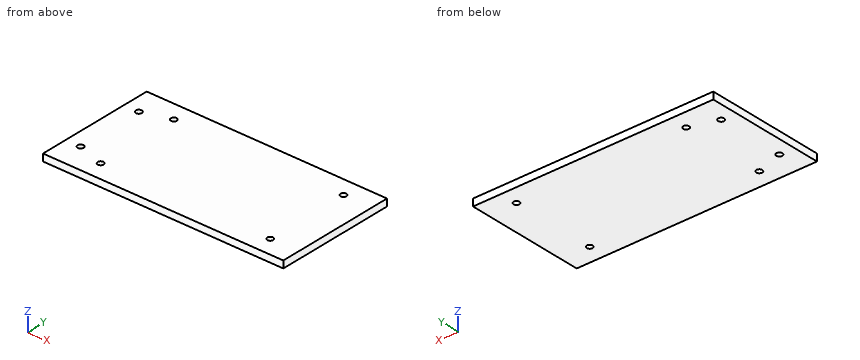
```python
from build123d import *

# Parameters (mm, degrees)
SKETCH1_W           = 85
SKETCH1_H           = 170
SKETCH1_R           = 2.1
BOSS_EXTRUDE1_DEPTH = 5
SKETCH2_R           = 2.15
CUT_EXTRUDE1_DEPTH  = 10
SKETCH3_R           = 2.15
CUT_EXTRUDE2_DEPTH  = 10


with BuildPart() as part:
    # Sketch1 → Boss-Extrude1 (new body)
    with BuildSketch(Plane(origin=(0, 0, 0), x_dir=(0, 1, 0), z_dir=(0, 0, 1))):
        Rectangle(SKETCH1_W, SKETCH1_H)
        with Locations(Location((-30, 55, 0), (0, 0, 270))):
            Circle(SKETCH1_R, mode=Mode.SUBTRACT)
        with Locations(Location((-30, -65, 0), (0, 0, 270))):
            Circle(SKETCH1_R, mode=Mode.SUBTRACT)
        with Locations(Location((30, -65, 0), (0, 0, 90))):
            Circle(SKETCH1_R, mode=Mode.SUBTRACT)
        with Locations(Location((30, 55, 0), (0, 0, 90))):
            Circle(SKETCH1_R, mode=Mode.SUBTRACT)
    extrude(amount=BOSS_EXTRUDE1_DEPTH)

    # Sketch2 → Cut-Extrude1 (cut)
    with BuildSketch(Plane(origin=(0, 0, 5), x_dir=(0, -1, 0), z_dir=(0, 0, 1))):
        with Locations(Location((23.85, -74.5, 0), (0, 0, 90))):
            Circle(SKETCH2_R)
    extrude(amount=-CUT_EXTRUDE1_DEPTH, mode=Mode.SUBTRACT)

    # Sketch3 → Cut-Extrude2 (cut)
    with BuildSketch(Plane(origin=(0, 0, 5), x_dir=(0, -1, 0), z_dir=(0, 0, 1))):
        with Locations(Location((-23.85, -74.5, 0), (0, 0, 90))):
            Circle(SKETCH3_R)
    extrude(amount=-CUT_EXTRUDE2_DEPTH, mode=Mode.SUBTRACT)


solid = part.part
```
Build history of the part. All positions in model axes, mm. Give positions to 0.01 mm unless a question says otherwise; leave off trailing zeros. Loops run counter-clockwise (first coordinate to the right, second up) from the corner with the lowest first, then second, coordinate; pieces in that order, holes last.
1) Probe line 1 along X through (y, z) = (30, 1.7); line 2 along Y through (x, z) = (65, 2.4); line 3 along Y through (x, z) = (-74.5, 1.75). List the from-to ranges inside material, lowest first.
Values follow:
line 1: x = -85 to -57.1, -52.9 to 62.9, 67.1 to 85
line 2: y = -42.5 to -32.1, -27.9 to 27.9, 32.1 to 42.5
line 3: y = -42.5 to -26, -21.7 to 21.7, 26 to 42.5
2) Band-saw the part on B-B on y = 30. List the corners of the cut face in (x, z).
Values follow:
outline: (-85, 0) - (-57.1, 0) - (-57.1, 5) - (-85, 5) - close; (-52.9, 0) - (62.9, 0) - (62.9, 5) - (-52.9, 5) - close; (67.1, 0) - (85, 0) - (85, 5) - (67.1, 5) - close
3) Drop a flat-ended pin along its axis: P1, Ø3.5, axis at x = 65, y = -30, coming from the -Z side. Give the stop position or say it passes through.
Values follow:
P1: passes through
4) Band-saw the part on A-A on x = 65. List the corners of the cut face in (y, z), then the cut area to 3 significant figures.
Values follow:
outline: (-42.5, 0) - (-32.1, 0) - (-32.1, 5) - (-42.5, 5) - close; (-27.9, 0) - (27.9, 0) - (27.9, 5) - (-27.9, 5) - close; (32.1, 0) - (42.5, 0) - (42.5, 5) - (32.1, 5) - close
area: 383 mm2
